from build123d import *

# Parameters (mm, degrees)
SKETCH3_W               = 60
SKETCH3_H               = 40
BOSS_EXTRUDE1_DEPTH     = 5
CUT_EXTRUDE1_DEPTH      = 73.284161474
CUT_EXTRUDE1_DEPTH_BACK = 73.284161474
SKETCH6_W               = 58
SKETCH6_H               = 38
SKETCH7_W               = 60
SKETCH7_H               = 40
BOSS_EXTRUDE2_DEPTH     = 1
CUT_EXTRUDE2_DEPTH      = 73.284161474
CUT_EXTRUDE2_DEPTH_BACK = 73.284161474
SKETCH8_W               = 50
SKETCH8_H               = 30


with BuildPart() as part:
    # Sketch3 → Boss-Extrude1 (new body)
    with BuildSketch(Plane(origin=(0, 0, 0), x_dir=(1, 0, 0), z_dir=(0, 1, 0))):
        with Locations((30, 20)):
            Rectangle(SKETCH3_W, SKETCH3_H)
    extrude(amount=BOSS_EXTRUDE1_DEPTH)

    # Sketch6 → Cut-Extrude1 (cut, two sides: drawn at the far end of the back side and taken through both)
    with BuildSketch(Plane(origin=(0, 0, 0), x_dir=(1, 0, 0), z_dir=(0, 1, 0)).offset(-CUT_EXTRUDE1_DEPTH_BACK)):
        with Locations((30, 20)):
            Rectangle(SKETCH6_W, SKETCH6_H)
    extrude(amount=CUT_EXTRUDE1_DEPTH + CUT_EXTRUDE1_DEPTH_BACK, mode=Mode.SUBTRACT)

    # Sketch7 → Boss-Extrude2 (add)
    with BuildSketch(Plane(origin=(0, 0, 0), x_dir=(1, 0, 0), z_dir=(0, 1, 0))):
        with Locations((30, 20)):
            Rectangle(SKETCH7_W, SKETCH7_H)
    extrude(amount=BOSS_EXTRUDE2_DEPTH)

    # Sketch8 → Cut-Extrude2 (cut, two sides: drawn at the far end of the back side and taken through both)
    with BuildSketch(Plane.XZ.offset(-CUT_EXTRUDE2_DEPTH_BACK)):
        with Locations((30, -20)):
            Rectangle(SKETCH8_W, SKETCH8_H)
    extrude(amount=CUT_EXTRUDE2_DEPTH + CUT_EXTRUDE2_DEPTH_BACK, mode=Mode.SUBTRACT)


solid = part.part
Model file for the job. Use its own axes, mm. A direction names the side the tool comes from. Give positions to 0.01 mm unless a question says otherwise; leave off trailing zeros. Write each loop counter-clockwise with the first axis right and the second up, starting at its lowest first coordinate (ties: lowest second). Pieces come first, ordered by that corner, then holes. Notation, with made-up numbers: (78, -32) -> (93, -32) arc R8 cw to (93, -19) -> close; hole circle Ø10 at (39, 65). An arc over 180 degrees is marked (long way). Write item = value, one per line.
(1) Slice it at B-B, the plane x = 15.5. Give the cut face in (y, z), then the cut area to 3 significant figures.
Determined:
outline = (0, -40) -> (5, -40) -> (5, -39) -> (1, -39) -> (1, -35) -> (0, -35) -> close; (0, -5) -> (1, -5) -> (1, -1) -> (5, -1) -> (5, 0) -> (0, 0) -> close
area = 18.0 mm2
(2) Slice it at C-C, the plane y = 2.75. Give the cut face in (x, z), then the cut area to 3 significant figures.
Determined:
outline = (0, -40) -> (60, -40) -> (60, 0) -> (0, 0) -> close; hole (1, -39) -> (59, -39) -> (59, -1) -> (1, -1) -> close
area = 196 mm2
(3) Mould opens along Z. For faces 1 (the face through (30, 3, -39)), 2 (the face through (30, 2, -40)), 3 (the face through (30, 3, -1)), 4 (the face through (30, 2, 0)) say: released by +Z, released by -Z, zero draft, split by the parting line, or undercut.
Determined:
face_1 = undercut
face_2 = released by -Z
face_3 = undercut
face_4 = released by +Z
(4) Slice it at D-D, the plane z = -3. Give the cut face in (x, y), then the cut area to 3 significant figures.
Determined:
outline = (0, 0) -> (60, 0) -> (60, 5) -> (59, 5) -> (59, 1) -> (1, 1) -> (1, 5) -> (0, 5) -> close
area = 68.0 mm2
(5) Slice it at A-A, the plane z = -15.5. Give the cut face in (x, y).
Determined:
outline = (0, 0) -> (5, 0) -> (5, 1) -> (1, 1) -> (1, 5) -> (0, 5) -> close; (55, 0) -> (60, 0) -> (60, 5) -> (59, 5) -> (59, 1) -> (55, 1) -> close
(6) Tool access for faces 5 (the face through (0, 2, -20)), 6 (the face through (30, 1, -3)): list every direction of +Z, -Z, +X, -X, +Y, -Y with a clear straight run to the whole face (end or side of a thin tool).
Determined:
face_5 = +Z, -Z, -X, +Y, -Y
face_6 = +Y
(7) Probe line 1 along X through (y, z) = (2.2, -36); line 2 along Z through (x, y) = (42, 4.85); line 3 along Z through (x, y) = (12.5, 0.5). List the from-to ranges inside material, lowest first.
Determined:
line_1 = 0 to 1, 59 to 60
line_2 = -40 to -39, -1 to 0
line_3 = -40 to -35, -5 to 0
